Read the model definition and answer for the solid it produces. Units are mm, in the model's axes. Face numbers are marked on the shaded views. A direction names the side the tool comes from. Coordinates: 2 decimals unless noted, no trailing zeros. Loops run counter-clockwise (first coordinate to the right, second up) from the corner with the lowest first, then second, coordinate; pieces in that order, holes last.
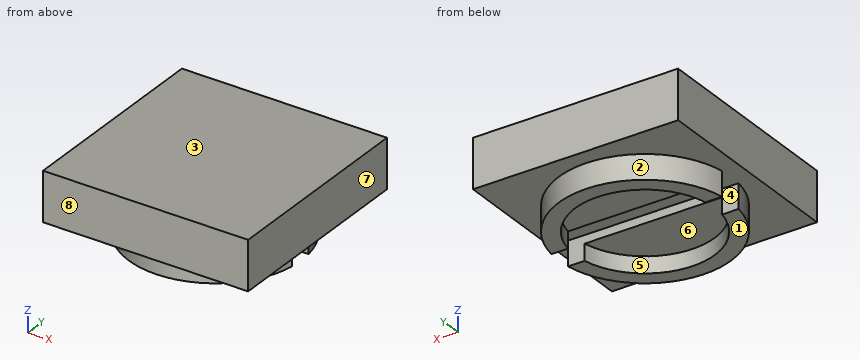
from build123d import *

# Parameters (mm, degrees)
F0_W          = 25
F0_H          = 25
F1_DEPTH      = 6
F2_R          = 10.5
F3_DEPTH      = 3
F4_R          = 8.5
F5_DEPTH      = 2
F6_W          = 3
F6_H          = 5
F7_DEPTH      = 25
F7_DEPTH_BACK = 25


with BuildPart() as f1:
    # F0 (on Top) → F1 (new body)
    with BuildSketch(Plane.XY):
        Rectangle(F0_W, F0_H)
    extrude(amount=F1_DEPTH)

    # F2 (on face) → F3 (join)
    with BuildSketch(Plane(origin=(0, 0, 0), x_dir=(1, 0, 0), z_dir=(0, 0, -1))):
        Circle(F2_R)
    extrude(amount=F3_DEPTH)

    # F4 (on face) → F5 (cut)
    with BuildSketch(Plane(origin=(0, 0, -3), x_dir=(1, 0, 0), z_dir=(0, 0, -1))):
        Circle(F4_R)
    extrude(amount=-F5_DEPTH, mode=Mode.SUBTRACT)

    # F6 (on Right) → F7 (cut, two sides)
    with BuildSketch(Plane.YZ) as f7_sk:
        with Locations((0, -2.5)):
            Rectangle(F6_W, F6_H)
    extrude(amount=-F7_DEPTH, mode=Mode.SUBTRACT)
    extrude(f7_sk.sketch, amount=F7_DEPTH_BACK, mode=Mode.SUBTRACT)


solid = f1.part
Q1. Determine the mould class of the marked faces 6, 7 and 8 for opening direction Y: +Y half, -Y half, draft (parallel to the pull), parting line (faces both ways), or undercut.
Findings below:
face 6: undercut
face 7: draft
face 8: -Y half
Q2. A cutting plane is placed at B-B (y = 5). Give the vertices of the cut face in (x, z), then the cut area to 3 significant figures.
Findings below:
outline: (-12.5, 0) - (-9.23, 0) - (-9.23, -3) - (-6.87, -3) - (-6.87, -1) - (6.87, -1) - (6.87, -3) - (9.23, -3) - (9.23, 0) - (12.5, 0) - (12.5, 6) - (-12.5, 6) - close
area: 178 mm2
Q3. Which of the six approach directions +Z, -Z, +X, -X, +Y, -Y give full straight-line access (tool end or side, diameter ignored) to the marked faces 1, 2, 3, 4 and 5?
Findings below:
face 1: -Z, +X, -X, +Y, -Y
face 2: -Z, +Y
face 3: +Z, +X, -X, +Y, -Y
face 4: -Z, +X, -X
face 5: -Z
Q4. A cutting plane is placed at D-D (y = 8). Give the vertices of the cut face in (x, z).
Findings below:
outline: (-12.5, 0) - (-6.8, 0) - (-6.8, -3) - (-2.87, -3) - (-2.87, -1) - (2.87, -1) - (2.87, -3) - (6.8, -3) - (6.8, 0) - (12.5, 0) - (12.5, 6) - (-12.5, 6) - close
Q5. A cutting plane is placed at C-C (x = 5). Give the vertices of the cut face in (y, z), then the cut area to 3 significant figures.
Findings below:
outline: (-12.5, 0) - (-9.23, 0) - (-9.23, -3) - (-6.87, -3) - (-6.87, -1) - (-1.5, -1) - (-1.5, 0) - (1.5, 0) - (1.5, -1) - (6.87, -1) - (6.87, -3) - (9.23, -3) - (9.23, 0) - (12.5, 0) - (12.5, 6) - (-12.5, 6) - close
area: 175 mm2
Q6. A cutting plane is placed at A-A (x = 1.5). Give the vertices of the cut face in (y, z).
Findings below:
outline: (-12.5, 0) - (-10.39, 0) - (-10.39, -3) - (-8.37, -3) - (-8.37, -1) - (-1.5, -1) - (-1.5, 0) - (1.5, 0) - (1.5, -1) - (8.37, -1) - (8.37, -3) - (10.39, -3) - (10.39, 0) - (12.5, 0) - (12.5, 6) - (-12.5, 6) - close
Q7. Straight lines are drawn through the part: probe 1 along Z at (x, y) = (9, -1); probe 2 along Z at (x, y) = (-6.5, -3.25); probe 3 along Y at (x, z) = (7.25, -2). For each, find the intervals that lie inside material, in ascending order.
Findings below:
probe 1: z = 0 to 6
probe 2: z = -1 to 6
probe 3: y = -7.6 to -4.44, 4.44 to 7.6
Q8. Flat-ended cylindrical pins translate along their axes: pin 1 Ø3.5 at (x, y) = (-1.5, -5.5) entering from -Z; pin 2 Ø2.5 at (x, z) = (-4, -2) entering from +Y. Find the tip coordinate at first contact, or state that the pin passes through.
Findings below:
pin 1: stops at z = -1
pin 2: stops at y = 10.13
